Can you work these out from the model? Positions are in its coordinate system, mm. A direction names the side the tool comes from. Coordinates: 2 decimals unless noted, no trailing zeros. Loops run counter-clockwise (first coordinate to the right, second up) from the corner with the lowest first, then second, coordinate; pieces in that order, holes last. Notation, with made-up numbers: (59.5, 53) -> (85.5, 53) arc R9 ccw to (85.5, 59) -> close; hole circle Ø5 at (51, -30). An arc over 180 degrees is marked (long way). Use one line per item in the form item = value. Start each with the question number.
(1) Imagine slicing it at A-A (z = 1.7). List the corners of the cut face in (x, y) for me, plus the area to 3 significant figures.
(2) I need wall thicknesses on line 1 (Y direction, x = 6, z = 4.85); line 2 (X direction, y = 9, z = 5.5); line 3 (X direction, y = 3, z = 4.55). Which ranges of each line are inside material? Lowest first, please. Write a range as [from, to].
(3) Imagine slicing it at C-C (x = 7.25). List the corners of the cut face in (y, z) for me, plus the area to 3 significant figures.
(4) Imagine slicing it at D-D (y = 2.5). List the corners of the cut face in (x, z) for me.
(5) Imagine slicing it at B-B (y = 5.5). List the corners of the cut face in (x, z) for me, plus the area to 3 significant figures.
(6) I'm going to push flat-ended pins straight in: pin 1 (0.9 mm diameter, centred on x = 1, y = 5, fed in from +Z); pin 2 (0.6 mm diameter, centred on y = 4, z = 5, fed in from -X); pin 3 (1 mm diameter, centred on y = 4.5, z = 5, fed in from +X). Where does each tip first touch, or does it pass through?
(7) Thinking about a two-plate mould opening in Y: for faces 1 (the flat face through (6, 0, 3)), 2 (the flat face through (9, 5, 5)), 3 (the cylindrical face through (6.99, 2.05, 2.99)), which applies, released by +Y, released by -Y, zero draft, split by the parting line, or undercut?
(8) On a 3-axis mill with a long thin cutter (end or side, diameter ignored), from which of +Z, -Z, +X, -X, +Y, -Y can I reach the whole of each face in a straight line? I mean faces 4 (the flat face through (1, 5, 3.9)), 5 (the flat face through (8, 5, 5.9)), 6 (the flat face through (10, 5, 3.9)). Say none if no direction works.
Autodesk Inventor part; units mm, degrees
ref_plane "YZ Plane" through (0, 0, 0) normal (1, 0, 0) x (0, 1, 0)
ref_plane "XZ Plane" through (0, 0, 0) normal (0, 1, 0) x (-1, 0, 0)
ref_plane "XY Plane" through (0, 0, 0) normal (0, 0, 1) x (1, 0, 0)
sketch "Skizze3" plane through (0, 0, 0) normal (0, 1, 0) x (-1, 0, 0)
  line L0 (0, 3.9) -> (-3, 3.9)
  line L1 (-3, 3.9) -> (-3, 5.9)
  line L2 (0, 3.9) -> (0, 3.1)
  line L3 (0, 3.1) -> (-3.1, 0)
  line L4 (-3, 5.9) -> (-5.7, 5.9)
  line L5 (-5.7, 5.9) -> (-6, 5.6)
  line L6 (-6, 5.6) -> (-6, 0)
  line L7 (-6, 0) -> (-3.1, 0)
  point P0 (0, 0)
  dimension "d6" = 3
  dimension "d7" = 6
  dimension "d8" = 3.1
  dimension "d9" = 5.9
  dimension "d10" = 135
  dimension "d11" = 0.3
  dimension "d12" = 2
  dimension "d13" = 135
extrude "Extrusion3" add sketch "Skizze3" along normal blind 10
mirror "Spiegeln1" about plane through (6, 0, 5.6) normal (1, 0, 0) of "Extrusion3"
sketch "Skizze4" plane through (3.1, 0, 0) normal (0, 0, -1) x (-1, 0, 0)
  line L0 (0, 0) -> (0, 10)
  line L1 (-5.8, 0) -> (-5.8, 10)
  line L2 (-2.9, 0) -> (-2.9, 10)
  line L3 (0, 10) -> (-5.8, 10)
  line L4 (0, 0) -> (-5.8, 0)
  point P0 (3.1, 0)
  point P1 (-2.9, 3.3333)
  dimension "d23" = 10
  dimension "d24" = 3.3333
hole "Bohrung1" at (6, 3.3333, 0) direction (0, 0, 1) diameter 3.242 end through all
properties part number "BTwnikel2_trajan20_21"
Worked out:
q1.outline = (1.4, 0) -> (10.6, 0) -> (10.6, 10) -> (1.4, 10) -> close; hole circle Ø3.24 at (6, 3.33)
q1.area = 83.7 mm2
q2.line_1 = [0, 1.71], [4.95, 10]
q2.line_2 = [3, 9]
q2.line_3 = [3, 4.41], [7.59, 9]
q3.outline = (0, 0) -> (2.3, 0) -> (2.3, 5.9) -> (0, 5.9) -> close; (4.37, 0) -> (10, 0) -> (10, 5.9) -> (4.37, 5.9) -> close
q3.area = 46.8 mm2
q4.outline = (0, 3.1) -> (3.1, 0) -> (4.61, 0) -> (4.61, 5.9) -> (3, 5.9) -> (3, 3.9) -> (0, 3.9) -> close; (7.39, 0) -> (8.9, 0) -> (12, 3.1) -> (12, 3.9) -> (9, 3.9) -> (9, 5.9) -> (7.39, 5.9) -> close
q5.outline = (0, 3.1) -> (3.1, 0) -> (8.9, 0) -> (12, 3.1) -> (12, 3.9) -> (9, 3.9) -> (9, 5.9) -> (6.3, 5.9) -> (6, 5.6) -> (5.7, 5.9) -> (3, 5.9) -> (3, 3.9) -> (0, 3.9) -> close
q5.area = 49.1 mm2
q6.pin_1 = 3.9
q6.pin_2 = 3
q6.pin_3 = 9
q7.face_1 = released by -Y
q7.face_2 = zero draft
q7.face_3 = undercut
q8.face_4 = +Z, -X, +Y, -Y
q8.face_5 = +Z, +X, -X, +Y, -Y
q8.face_6 = +Z, +X, +Y, -Y
